from build123d import *

# Parameters (mm, degrees)
SKETCH_W        = 14
SKETCH_H        = 8.5
PAD_DEPTH       = 0.5
SKETCH001_R     = 0.625
POCKET_DEPTH    = 0.501
SKETCH002_R     = 2.5
PAD001_DEPTH    = 2
SKETCH003_R     = 1.55
POCKET001_DEPTH = 2.501
FILLET_R        = 0.5


with BuildPart() as part:
    # Sketch → Pad (new body)
    with BuildSketch(Plane.XY):
        Rectangle(SKETCH_W, SKETCH_H)
    extrude(amount=PAD_DEPTH)

    # Sketch001 (on Face6 of Pad) → Pocket (cut, through all)
    with BuildSketch(Plane.XY.offset(0.5)):
        with Locations((-5.625, 2.625)):
            Circle(SKETCH001_R)
        with Locations((5.625, -2.625)):
            Circle(SKETCH001_R)
    extrude(amount=-POCKET_DEPTH, mode=Mode.SUBTRACT)

    # Sketch002 (on Face5 of Pocket) → Pad001 (join)
    with BuildSketch(Plane.XY.offset(0.5)):
        Circle(SKETCH002_R)
    extrude(amount=PAD001_DEPTH)

    # Sketch003 (on Face10 of Pad001) → Pocket001 (cut, through all)
    with BuildSketch(Plane.XY.offset(2.5)):
        Circle(SKETCH003_R)
    extrude(amount=-POCKET001_DEPTH, mode=Mode.SUBTRACT)

    # Fillet
    fillet_edges = [part.edges().sort_by_distance(p)[0] for p in [
        (-7, -4.25, 0.25),
        (7, -4.25, 0.25),
        (7, 4.25, 0.25),
        (-7, 4.25, 0.25),
    ]]
    fillet(fillet_edges, radius=FILLET_R)


solid = part.part
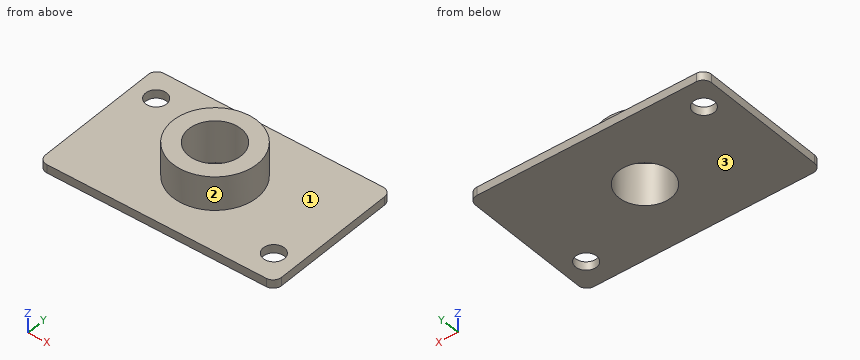
Verification items for the finished model (mm, model axes). Face numbers are marked on the shaded views. Coordinates: 2 decimals unless noted, no trailing zeros. Order: outer loops, then holes, each group sorted by start corner. A loop starts at its lowest first (then second) coordinate and runs counter-clockwise, first axis right, second up.
1. Scan lines: line 1 (Z direction, x = 3, y = -1); line 2 (X direction, y = -3, z = 0.4) (3 decimals); line 3 (X direction, y = -1.25, z = 2.3). Record each from-to range of solid material in increasing order.
Results found:
line 1: z = 0 to 0.5
line 2: x = -7 to 5.125, 6.125 to 7
line 3: x = -2.17 to -0.92, 0.92 to 2.17
2. Sectioned sample at D-D, the plane z = 0.7. Record the cut outline in (x, y).
Results found:
outline: circle Ø5 at (0, 0); hole circle Ø3.1 at (0, 0)
3. Sectioned sample at C-C, the plane x = 4. Record the cut outline in (y, z).
Results found:
outline: (-4.25, 0) - (4.25, 0) - (4.25, 0.5) - (-4.25, 0.5) - close
4. Go/stop test with a flat-tipped pin: pin 1 Ø3 at (x, y) = (0, 0) entering from -Z. Record where the tip stops, or that it passes through.
Results found:
pin 1: passes through
5. Release check for a two-part mould opening along Z. For the marked faces 1, 2 and 3 record: +Z half, -Z half, draft (parallel to the pull), parting line (faces both ways), or undercut.
Results found:
face 1: +Z half
face 2: draft
face 3: -Z half
6. Sectioned sample at B-B, the plane x = 0. Record the cut outline in (y, z), and give its area (3 significant figures).
Results found:
outline: (-4.25, 0) - (-1.55, 0) - (-1.55, 2.5) - (-2.5, 2.5) - (-2.5, 0.5) - (-4.25, 0.5) - close; (1.55, 0) - (4.25, 0) - (4.25, 0.5) - (2.5, 0.5) - (2.5, 2.5) - (1.55, 2.5) - close
area: 6.50 mm2
7. Sectioned sample at A-A, the plane y = 0. Record the cut outline in (x, z), and give its area (3 significant figures).
Results found:
outline: (-7, 0) - (-1.55, 0) - (-1.55, 2.5) - (-2.5, 2.5) - (-2.5, 0.5) - (-7, 0.5) - close; (1.55, 0) - (7, 0) - (7, 0.5) - (2.5, 0.5) - (2.5, 2.5) - (1.55, 2.5) - close
area: 9.25 mm2
